Part model, mm, in its own coordinate system. A direction names the side the tool comes from. Give positions to 0.01 mm unless a question says otherwise; leave off trailing zeros. Write each loop counter-clockwise with the first axis right and the second up, starting at its lowest first coordinate (ties: lowest second). Pieces come first, ordered by that corner, then holes.
```python
from build123d import *

# Parameters (mm, degrees)
SKETCH1_W           = 60
SKETCH1_H           = 40
BOSS_EXTRUDE1_DEPTH = 22
SKETCH2_W           = 60
SKETCH2_H           = 5.1
SKETCH2_H_2         = 8
CUT_EXTRUDE1_DEPTH  = 15
FILLET1_R           = 10
SKETCH3_W           = 60
SKETCH3_H           = 7
BOSS_EXTRUDE2_DEPTH = 10


with BuildPart() as part:
    # Sketch1 → Boss-Extrude1 (new body)
    with BuildSketch(Plane(origin=(0, 0, 0), x_dir=(1, 0, 0), z_dir=(0, 1, 0))):
        Rectangle(SKETCH1_W, SKETCH1_H)
    extrude(amount=BOSS_EXTRUDE1_DEPTH)

    # Sketch2 → Cut-Extrude1 (cut)
    with BuildSketch(Plane(origin=(0, 22, 0), x_dir=(1, 0, 0), z_dir=(0, 1, 0))):
        Rectangle(SKETCH2_W, SKETCH2_H)
        with Locations((0, 16)):
            Rectangle(SKETCH2_W, SKETCH2_H_2)
        with Locations((0, -16)):
            Rectangle(SKETCH2_W, SKETCH2_H_2)
    extrude(amount=-CUT_EXTRUDE1_DEPTH, mode=Mode.SUBTRACT)

    # Fillet1
    # the kernel refuses this fillet: 10 mm, written as the material it adds along each edge
    with BuildSketch(Plane(origin=(-30, 7, 12), x_dir=(0, 0, 1), z_dir=(1, 0, 0)), Plane(origin=(30, 7, -12), x_dir=(0, 0, -1), z_dir=(-1, 0, 0))) as fillet1_piece_1:
        with BuildLine():
            CenterArc((10, -9.797958971), FILLET1_R, 101.536959033, 78.463040967)
            Line((0, -9.797958971), (-0.2, -9.797958971))
            Line((-0.2, -9.797958971), (-0.2, 0))
            Line((-0.2, 0), (0, 0.2))
            ThreePointArc((0, 0.2), (4, 0.2), (7.96, 0.195959179))
            Line((7.96, 0.195959179), (8, 0))
        make_face()
    extrude(amount=60)

    # Sketch3 → Boss-Extrude2 (add)
    with BuildSketch(Plane.XY.offset(20)):
        with Locations((0, 3.5)):
            Rectangle(SKETCH3_W, SKETCH3_H)
    extrude(amount=BOSS_EXTRUDE2_DEPTH)


solid = part.part
```
1) Pin check, flat tips, straight feed: pin 1 Ø11 at (x, z) = (9, 26.5) entering from +Y; pin 2 Ø4.5 at (x, y) = (-13.5, 16.5) entering from +Z; pin 3 Ø4.5 at (x, y) = (-11.5, 14.5) entering from -Z; pin 4 Ø1 at (x, z) = (13.5, 7) entering from -Y. Stop position of each tip, or through.
Answers follow:
pin 1: stops at y = 7
pin 2: stops at z = 12.33
pin 3: stops at z = -13.09
pin 4: stops at y = 0
2) Saw through at D-D, the plane z = 25. Write the cut outline in (x, y), then the cut area to 3 significant figures.
Answers follow:
outline: (-30, 0) - (30, 0) - (30, 7) - (-30, 7) - close
area: 420 mm2
3) 3-axis set-ups, long thin cutter, end or side, ignore diameter. For faces 1 (the face through (0, 7, 0)), 2 (the face through (0, 19, 12)), 3 (the face through (30, 8, 5)): which of +Z, -Z, +X, -X, +Y, -Y reach the whole face in a straight line?
Answers follow:
face 1: +X, -X, +Y
face 2: +Z, +X, -X, +Y
face 3: +Z, -Z, +X, +Y, -Y
4) Wall check: L1, parallel to Z at x = 0, y = 16.75; L2, parallel to Y at x = 24, z = 24; L3, parallel to Z at x = 1, y = 10. Give the ranges that are in metal, low to high.
Answers follow:
L1: z = -12 to -2.55, 2.55 to 12
L2: y = 0 to 7
L3: z = -14.67 to -2.55, 2.55 to 14.67
5) Saw through at A-A, the plane y = 18. Write the cut outline in (x, z).
Answers follow:
outline: (-30, -12) - (30, -12) - (30, -2.55) - (-30, -2.55) - close; (-30, 2.55) - (30, 2.55) - (30, 12) - (-30, 12) - close
6) Saw through at C-C, the plane y = 11.5. Write the cut outline in (x, z), then the cut area to 3 significant figures.
Answers follow:
outline: (-30, -13.52) - (30, -13.52) - (30, -2.55) - (-30, -2.55) - close; (-30, 2.55) - (30, 2.55) - (30, 13.52) - (-30, 13.52) - close
area: 1,320 mm2
7) Two-plate mould, pull along Z, no slides. Class faces 4 (the face through (0, 15, -2.55)), 5 (the face through (0, 19, -12)), 6 (the face through (0, 4, 30)): +Z half, -Z half, draft (parallel to the pull), parting line (faces both ways), or undercut.
Answers follow:
face 4: undercut
face 5: -Z half
face 6: +Z half
8) Saw through at B-B, the plane x = 19. Write the cut outline in (y, z), then the cut area to 3 significant figures.
Answers follow:
outline: (0, -20) - (7, -20) arc R10 cw to (16.8, -12) - (22, -12) - (22, -2.55) - (7, -2.55) - (7, 2.55) - (22, 2.55) - (22, 12) - (16.8, 12) arc R10 cw to (7, 20) - (7, 30) - (0, 30) - close
area: 673 mm2
